```python
from build123d import *

# Parameters (mm, degrees)
F1_DEPTH        = 15.875
F2_W            = 15.875
F2_H            = 15.875
F3_DEPTH        = 76.2
F6_W            = 105.9110574424
F6_H            = 138.153988868
F7_DEPTH        = 12.8143632709
F20_DEPTH       = 15.875
F22_DEPTH       = 15.875
F24_D           = 4.4958
F24_DEPTH       = 15.875
F24_CSINK_D     = 9.1186
F24_CSINK_ANGLE = 82
F24_TIP         = 1.3506745855


with BuildPart() as f1:
    # F0 (on Top) → F1 (new body)
    with BuildSketch(Plane.XY):
        Polygon((-15.875, 0), (0, 0), (53.975, 0), (53.975, 15.875), (0, 15.875), (0, 69.85), (-15.875, 69.85), align=None)
    extrude(amount=F1_DEPTH)

    # F2 (on face) → F3 (join)
    with BuildSketch(Plane(origin=(0, 0, 0), x_dir=(1, 0, 0), z_dir=(0, 0, -1))):
        with Locations((-7.9375, -7.9375)):
            Rectangle(F2_W, F2_H)
    extrude(amount=F3_DEPTH)

    # F6 (on face) → F7 (cut, through all)
    with BuildSketch(Plane(origin=(-0.3578752004, -0.3578752004, 0.0711293976), x_dir=(-0.6867913388, 0.7139219677, 0.1365030439), z_dir=(0.7002252666, 0.7002252666, -0.139173101))):
        with Locations((-0.5843583494, -35.3862922639)):
            Rectangle(F6_W, F6_H)
    extrude(amount=-F7_DEPTH, mode=Mode.SUBTRACT)

    # F9 (on face) → F10 section 0
    with BuildSketch(Plane(origin=(0, 0, 0), x_dir=(1, 0, 0), z_dir=(0, 0, -1)), mode=Mode.PRIVATE) as f10_s0:
        Polygon((0, -28.575), (0, -15.875), (-15.875, -15.875), align=None)
    loft([f10_s0.sketch, Vertex(-15.875, 15.875, -76.2)])

    # F11 (on face) → F12 section 0
    with BuildSketch(Plane(origin=(0, 0, 0), x_dir=(1, 0, 0), z_dir=(0, 0, -1)), mode=Mode.PRIVATE) as f12_s0:
        Polygon((0, 0), (0, -15.875), (12.7, -15.875), align=None)
    loft([f12_s0.sketch, Vertex(0, 0, -76.2)])

    # F13 (on face) → F14 section 0
    with BuildSketch(Plane(origin=(0, 0, 0), x_dir=(1, 0, 0), z_dir=(0, 0, -1)), mode=Mode.PRIVATE) as f14_s0:
        Polygon((12.7, -15.875), (0, -15.875), (0, -28.575), align=None)
    loft([f14_s0.sketch, Vertex(0, 15.875, 15.875)])

    # F15 (on face) → F16 section 0
    with BuildSketch(Plane(origin=(0, 0, -76.2), x_dir=(1, 0, 0), z_dir=(0, 0, -1)), mode=Mode.PRIVATE) as f16_s0:
        Polygon((0, -15.875), (0, 0), (-15.875, -15.875), align=None)
    loft([f16_s0.sketch, Vertex(0, 15.875, 0)], mode=Mode.SUBTRACT)

    # F14_face (on face) → F18 section 0
    with BuildSketch(Plane(origin=(4.2333333333, 20.1083333333, 0), x_dir=(1, 0, 0), z_dir=(0, 0, -1))):
        Polygon((8.4666666667, 4.2333333333), (-4.2333333333, 4.2333333333), (-4.2333333333, -8.4666666667), align=None)
    # F3_face (on face) → F18 section 1
    with BuildSketch(Plane(origin=(-7.9375, 7.9375, -76.2), x_dir=(1, 0, 0), z_dir=(0, 0, -1))):
        Polygon((-7.9375, -7.9375), (7.9375, 7.9375), (-7.9375, 7.9375), align=None)
    loft()

    # F19 (on face) → F20 (cut, through all)
    with BuildSketch(Plane(origin=(-15.875, 0, 0), x_dir=(0, -1, 0), z_dir=(-1, 0, 0))):
        Polygon((-69.85, 14.2875), (-69.85, 0), (-55.5498, 0), align=None)
    extrude(amount=-F20_DEPTH, mode=Mode.SUBTRACT)

    # F21 (on face) → F22 (cut, through all)
    with BuildSketch(Plane.XZ):
        Polygon((39.6875, 0), (53.975, 0), (53.975, 14.2875), align=None)
    extrude(amount=-F22_DEPTH, mode=Mode.SUBTRACT)

    # F24
    with Locations(Plane(origin=(0, 0, 0), x_dir=(1, 0, 0), z_dir=(0, 0, -1))):
        with Locations((-7.9375, -42.8498), (26.9875, -7.9375)):
            CounterSinkHole(F24_D / 2, F24_CSINK_D / 2, depth=F24_DEPTH, counter_sink_angle=F24_CSINK_ANGLE)
            with Locations((0, 0, -(F24_DEPTH + F24_TIP / 2))):  # 118° drill point
                Cone(0, F24_D / 2, F24_TIP, mode=Mode.SUBTRACT)


solid = f1.part
```
The model under review builds one solid part; all positions refer to its coordinate system, in mm. A direction names the side the tool comes from. Round coordinates to 2 decimals unless told otherwise and drop trailing zeros. Loops run counter-clockwise (first coordinate to the right, second up) from the corner with the lowest first, then second, coordinate; pieces in that order, holes last. Notation, with made-up numbers: M 0.25,89.25 L 52.25,89.25 A12 ccw 52.25,93.25 Z; hole C 12,80 d1. An arc over 180 degrees is marked long. Put each result on its own line as item: value.
Q1. Consider section A-A, the plane y = 51.5. Give the boundary of the cut face in (x, z) (3 decimals), then the cut area to 3 significant figures.
Result set:
outline: M -15.875,0 L 0,0 L 0,15.875 L -15.875,15.875 Z
area: 252 mm²
Q2. Machinability: for faces 5 (the flat face through (0, 42, 10)), 6 (the flat face through (-2, 22, 15.875)), 7 (the flat face through (4, 5, -22)), which of the approach directions +Z, -Z, +X, -X, +Y, -Y give a long, thin tool a straight path to every point of the face, cutting with its end or side? Answer none if there is none.
Result set:
face 5: +Z, +X, +Y
face 6: +Z, +X, -X, +Y, -Y
face 7: -Z, +X, -Y
Q3. Consider section B-B, the plane x = 21. Give the boundary of the cut face in (y, z) (3 decimals), then the cut area to 3 significant figures.
Result set:
outline: M 0,0 L 15.875,0 L 15.875,15.875 L 0,15.875 Z
area: 252 mm²
Q4. Mouldability with a two-part tool opening along X and no side actions: class faces 1 (the flat face through (-11.58, 19.31, -21.7)), 2 (the cylindrical face through (27.28, 5.71, 9.36)), 3 (the flat face through (-8, 36, 0)), 4 (the flat face through (46.93, 7.83, 7.24)) as released by +X, released by -X, zero draft, split by the parting line, or undercut.
Result set:
face 1: released by -X
face 2: undercut
face 3: zero draft
face 4: released by +X
Q5. For pin 1 (12 mm diameter, centred on y = 27, z = -15, fed in from +X); pin 2 (7 mm diameter, centred on x = 26.99, y = 7.94, fed in from +Z) (3 decimals); pin 3 (17.5 mm diameter, centred on x = 14, z = 6.5, fed in from +Y); pin 4 (5 mm diameter, centred on x = 14, y = 4.5, fed in from -Z), all flat-tipped, find the tip position at first contact; note any pin that passes through.
Result set:
pin 1: stops at x = 2.36
pin 2: stops at z = 15.875
pin 3: stops at y = 20.58
pin 4: stops at z = 0
Q6. To check wall thickness, follow L1, parallel to Y at x = 25, z = 11 (3 decimals); L2, parallel to Y at x = -1, z = -45; L3, parallel to Z at x = 34, y = 11.5 (3 decimals). State the ranges of each line that lie inside material, in increasing order.
Result set:
L1: y = 0 to 6.887, 8.988 to 15.875
L2: y = 0 to 12.7
L3: z = 0 to 15.875
